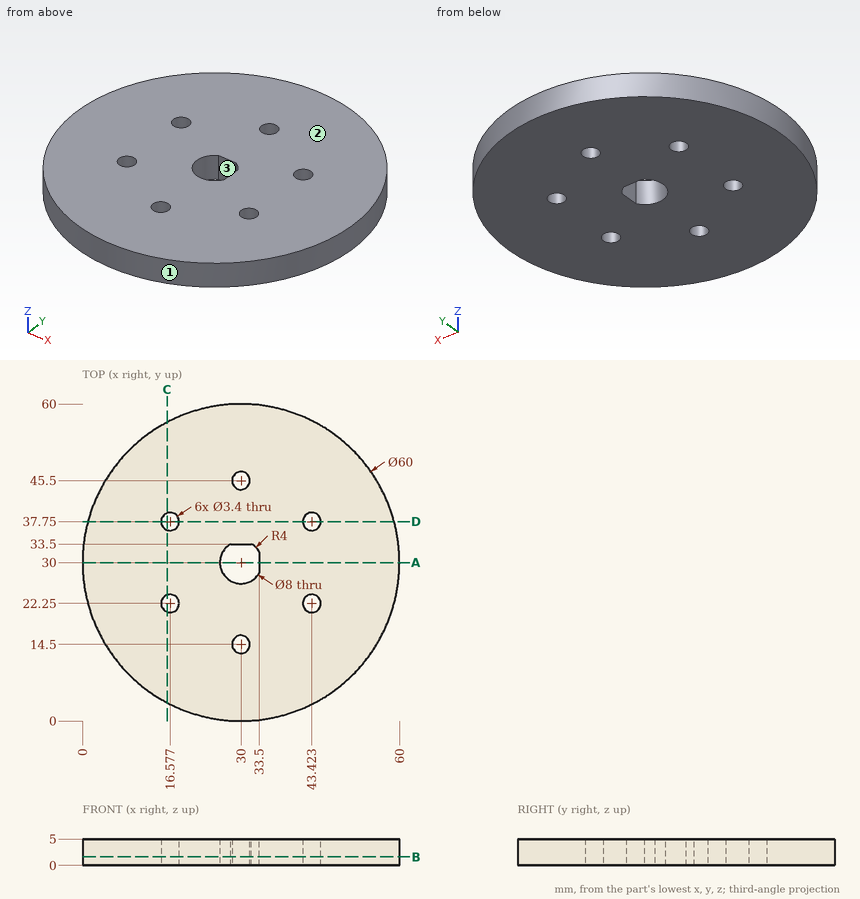
Design review of the part shown in the three views and the two pictorial views. Dimensions are in mm from the part's minimum x, y and z. Give positions to 0.01 mm unless a question says otherwise; leave off trailing zeros. Loops run counter-clockwise (first coordinate to the right, second up) from the corner with the lowest first, then second, coordinate; pieces in that order, holes last. Notation, with made-up numbers: (-23.5, 60.5) -> (15.5, 60.5) arc R21 cw to (15.5, 88.5) -> close; hole circle Ø11 at (-7, 73). An arc over 180 degrees is marked (long way). Answer as a JSON object with one key per item and string values. Group by question number.
Q1. Wall thickness on line 1 along Y through (x, z) = (31.5, 2.15) (1 decimal); line 2 along X through (y, z) = (37, 4.85); line 3 along X through (y, z) = (14, 2.1) (1 decimal): over which ranges is each line inside the solid? List them lowest first.
Q2. Insertion check: pin 1 (2 mm diameter, centred on x = 16.58, y = 37.75, fed in from +Z); pin 2 (3 mm diameter, centred on x = 30.5, z = 2.5, fed in from -Y); pin 3 (2 mm diameter, centred on x = 53.5, z = 4.5, fed in from -Y). Each pin has a flat end and moves straight along its axis. Give the tip position at first contact, or say it passes through.
Q3. Take a section at D-D (y = 37.75). Write out the cut boundary in (x, z), plus the area to 3 significant figures.
Q4. Take a section at B-B (z = 1.6). Write out the cut boundary in (x, y), plus the area to 3 significant figures.
Q5. Take a section at C-C (x = 16). Write out the cut boundary in (y, z).
Q6. Take a section at A-A (y = 30). Write out the cut boundary in (x, z).
Q7. Draft analysis for pull direction Y (two halves, no side actions). For the marked faces 1, 2 and 3, state which applies: pulls with the +Y half, pulls with the -Y half, needs draft (parallel to the pull), parting line crosses it, or undercut.
Answer below:
{
 "1": {"line 1": "y = 0 to 13.7, 15.3 to 26.3, 33.5 to 44.7, 46.3 to 60", "line 2": "x = 0.83 to 15.05, 18.1 to 41.9, 44.95 to 59.17", "line 3": "x = 4.6 to 28.4, 31.6 to 55.4"},
 "2": {"pin 1": "passes through", "pin 2": "stops at y = 0", "pin 3": "stops at y = 10.16"},
 "3": {"outline": "(1.02, 0) -> (14.88, 0) -> (14.88, 5) -> (1.02, 5) -> close; (18.28, 0) -> (41.72, 0) -> (41.72, 5) -> (18.28, 5) -> close; (45.12, 0) -> (58.98, 0) -> (58.98, 5) -> (45.12, 5) -> close", "area": "256 mm2"},
 "4": {"outline": "circle Ø60 at (30, 30); hole circle Ø3.4 at (16.58, 22.25); hole circle Ø3.4 at (16.58, 37.75); hole (28.06, 33.5) arc R4 ccw (long way) to (33.5, 28.06) -> (33.5, 31.94) arc R4 ccw to (31.94, 33.5) -> close; hole circle Ø3.4 at (30, 14.5); hole circle Ø3.4 at (30, 45.5); hole circle Ø3.4 at (43.42, 22.25); hole circle Ø3.4 at (43.42, 37.75)", "area": "2,730 mm2"},
 "5": {"outline": "(3.47, 0) -> (20.65, 0) -> (20.65, 5) -> (3.47, 5) -> close; (23.85, 0) -> (36.15, 0) -> (36.15, 5) -> (23.85, 5) -> close; (39.35, 0) -> (56.53, 0) -> (56.53, 5) -> (39.35, 5) -> close"},
 "6": {"outline": "(0, 0) -> (26, 0) -> (26, 5) -> (0, 5) -> close; (33.5, 0) -> (60, 0) -> (60, 5) -> (33.5, 5) -> close"},
 "7": {"face 1": "parting line crosses it", "face 2": "needs draft", "face 3": "undercut"}
}
